Geometry: see drawing. Coordinates: mm, zero at the bounding-box minimum. Coordinates: 2 decimals unless noted, no trailing zeros. Write each loop counter-clockwise with the first axis right and the second up, starting at its lowest first coordinate (ties: lowest second). Pieces come first, ordered by that corner, then holes. Notation, with made-up numbers: (-36, -31) - (5, -31) arc R6 cw to (5, -23) - close; hole circle Ø7 at (13.5, 22). An arc over 180 degrees is marked (long way). One line per question, with ' | ' between items. Start each with the question number.
Q1. Contact query for a flat-ended pin moving along its axis: P1, Ø8, axis at x = 29, y = 34.67, coming from the -Z side. Output: stop coordinate, or through.
Q2. Cut plane B-B, the plane y = 112. Return loops of the section in (x, z), plus the area to 3 significant figures.
Q3. Line query: line 1 (X direction, y = 76, z = 7.5); line 2 (Y direction, x = 60.5, z = 5); line 3 (Y direction, x = 6.5, z = 6.75). Output: solid intervals per line, ascending.
Q4. Cut plane D-D, the plane y = 84. Return loops of the section in (x, z).
Q5. Cut plane A-A, the plane x = 92. Return loops of the section in (y, z), plus the area to 3 significant figures.
Q6. Cut plane C-C, the plane z = 1.5. Give the number of separate pieces and of enclosed holes in the cut face, plus the area to 3 significant figures.
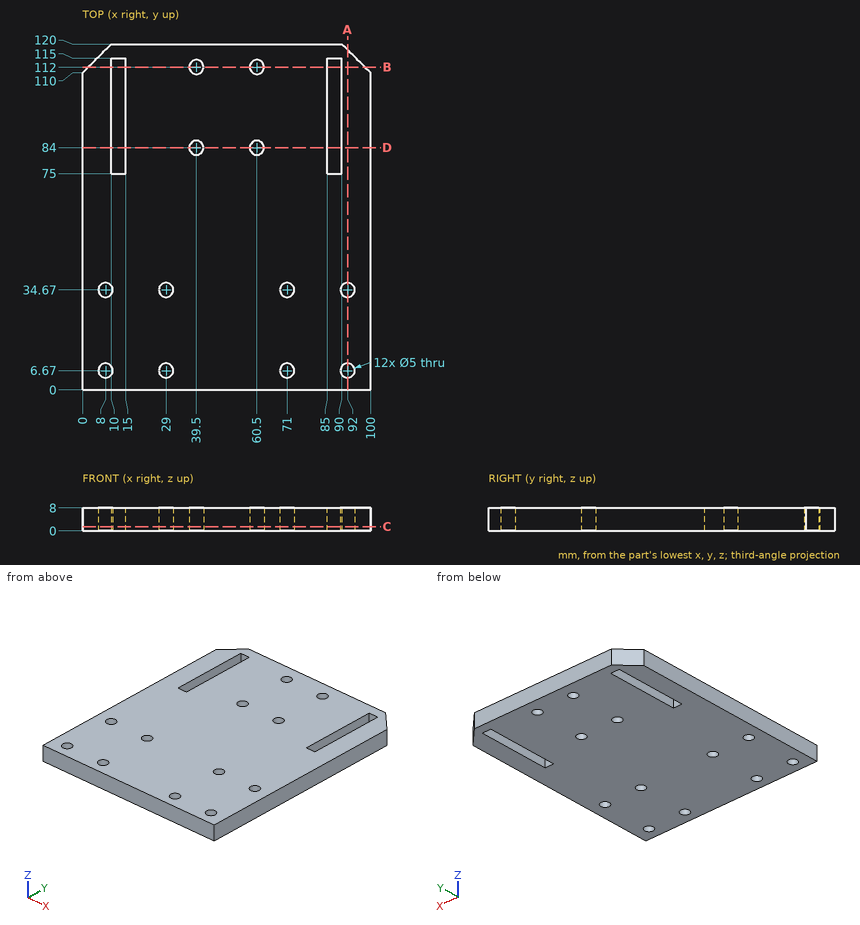
Reply:
1) P1: stops at z = 0
2) outline: (2, 0) - (10, 0) - (10, 8) - (2, 8) - close; (15, 0) - (37, 0) - (37, 8) - (15, 8) - close; (42, 0) - (58, 0) - (58, 8) - (42, 8) - close; (63, 0) - (85, 0) - (85, 8) - (63, 8) - close; (90, 0) - (98, 0) - (98, 8) - (90, 8) - close | area: 608 mm^2
3) line 1: x = 0 to 10, 15 to 85, 90 to 100 | line 2: y = 0 to 81.5, 86.5 to 109.5, 114.5 to 120 | line 3: y = 0 to 4.67, 8.67 to 32.67, 36.67 to 116.5
4) outline: (0, 0) - (10, 0) - (10, 8) - (0, 8) - close; (15, 0) - (37, 0) - (37, 8) - (15, 8) - close; (42, 0) - (58, 0) - (58, 8) - (42, 8) - close; (63, 0) - (85, 0) - (85, 8) - (63, 8) - close; (90, 0) - (100, 0) - (100, 8) - (90, 8) - close
5) outline: (0, 0) - (4.17, 0) - (4.17, 8) - (0, 8) - close; (9.17, 0) - (32.17, 0) - (32.17, 8) - (9.17, 8) - close; (37.17, 0) - (118, 0) - (118, 8) - (37.17, 8) - close | area: 864 mm^2
6) separate pieces: 1 | enclosed holes: 14 | area: 11,300 mm^2
